```python
from build123d import *

# Parameters (mm, degrees)
F0_W        = 45.5
F0_H        = 83.5
F1_DEPTH    = 52
F2_W        = 34
F2_H        = 72
F3_DEPTH    = 52.001
F5_W        = 15
F5_H        = 2
F6_DEPTH    = 52.001
F8_R        = 2
F10_D       = 4.4
F10_ON_F9_D = 4.4
F10_ON_F4_D = 4.4
F12_DEPTH   = 45.501
F13_W       = 7
F13_H       = 10
F14_DEPTH   = 2.5
F15_W       = 7.7
F15_H       = 31.3
F16_DEPTH   = 2.5


# Not quite as in the source:
# - a feature names something its author has since deleted; it is built from what else it names


with BuildPart() as f1:
    # F0 (on Front) → F1 (new body)
    with BuildSketch(Plane.XZ):
        with Locations((11.25, 30.25)):
            Rectangle(F0_W, F0_H)
    extrude(amount=F1_DEPTH)

    # F2 (on face) → F3 (cut, through all)
    with BuildSketch(Plane.XZ.offset(52)):
        with Locations((17, 36)):
            Rectangle(F2_W, F2_H)
    extrude(amount=-F3_DEPTH, mode=Mode.SUBTRACT)

    # F5 (on face) → F6 (cut, through all)
    with BuildSketch(Plane.XZ.offset(52)):
        with Locations((26.5, -10.5)):
            Rectangle(F5_W, F5_H)
    extrude(amount=-F6_DEPTH, mode=Mode.SUBTRACT)

    # F8
    f8_edges = [f1.edges().sort_by_distance(p)[0] for p in [
        (0, -26, 0),
    ]]
    fillet(f8_edges, radius=F8_R)

    # F10 (through all)
    with Locations(Plane.XY):
        with Locations((26.5, -4.2)):
            Hole(F10_D / 2)

    # F10 on F9 (through all)
    with Locations(Plane(origin=(-11.5, 0, 0), x_dir=(0, -1, 0), z_dir=(-1, 0, 0))):
        with Locations((12.2, 32.3)):
            Hole(F10_ON_F9_D / 2)

    # F10 on F4 (through all)
    with Locations(Plane(origin=(0, 0, -11.5), x_dir=(1, 0, 0), z_dir=(0, 0, -1))):
        with Locations((14.3, 19.8), (14.3, 4.2)):
            Hole(F10_ON_F4_D / 2)

    # F11 (on face) → F12 (cut, through all)
    with BuildSketch(Plane(origin=(-11.5, 0, 0), x_dir=(0, -1, 0), z_dir=(-1, 0, 0))):
        with BuildLine():
            ThreePointArc((47.8, 70), (46.2443650814, 69.3556349186), (45.6, 67.8))
            Line((45.6, 67.8), (45.6, 44.2))
            ThreePointArc((45.6, 44.2), (46.2443650814, 42.6443650814), (47.8, 42))
            ThreePointArc((47.8, 42), (49.3556349186, 42.6443650814), (50, 44.2))
            Line((50, 44.2), (50, 67.8))
            ThreePointArc((50, 67.8), (49.3556349186, 69.3556349186), (47.8, 70))
        make_face()
    extrude(amount=-F12_DEPTH, mode=Mode.SUBTRACT)

    # F13 (on face) → F14 (cut)
    with BuildSketch(Plane.YZ):
        with Locations((-12.2, 32.3)):
            Rectangle(F13_W, F13_H)
    extrude(amount=-F14_DEPTH, mode=Mode.SUBTRACT)

    # F15 (on face) → F16 (cut)
    with BuildSketch(Plane.YZ):
        with Locations((-48.15, 56.35)):
            Rectangle(F15_W, F15_H)
        with BuildLine():
            Line((-50, 44.2), (-50, 67.8))
            ThreePointArc((-50, 67.8), (-47.8, 70), (-45.6, 67.8))
            Line((-45.6, 67.8), (-45.6, 44.2))
            ThreePointArc((-45.6, 44.2), (-47.8, 42), (-50, 44.2))
        make_face(mode=Mode.SUBTRACT)
    extrude(amount=-F16_DEPTH, mode=Mode.SUBTRACT)


solid = f1.part
```
CAD build for the part. Positions are in the model's coordinates, mm. A direction names the side the tool comes from. Coordinates: 2 decimals unless noted, no trailing zeros. Loops run counter-clockwise (first coordinate to the right, second up) from the corner with the lowest first, then second, coordinate; pieces in that order, holes last. Notation, with made-up numbers: (40.5, -20) - (83.5, -20) arc R17 ccw to (83.5, 7) - close; hole circle Ø1 at (-4, 22.25). An arc over 180 degrees is marked (long way). Use CSV: the item, a comma, the result in double quotes. Start each with the question number.
Q1. Cut at A-A, the plane y = -12.2. List the corners of the cut face in (x, z).
Q2. Cut at B-B, the plane x = 26.5. List the corners of the cut face in (y, z), then the cut area to 3 significant figures.
Q3. Probe probe 1 along Y at (x, z) = (14.3, -2.5); probe 2 along Y at (x, z) = (-4, 32); probe 3 along Z at (x, y) = (-4, -12). List the from-to ranges inside material, lowest first. Write a range as from..to.
Q4. Cut at D-D, the plane x = 14.3. List the corners of the cut face in (y, z), then the cut area to 3 significant figures.
Q5. Two-plate mould, pull along Y, no slides. Class faces 1 (the cylindrical face through (0.57, -25.64, 0.6)), 2 (the flat face through (-1, -12, 27.3)), 3 (the flat face through (-2, 0, 21)): +Y half, -Y half, draft (parallel to the pull), parting line (faces both ways), or undercut.
Q6. 3-axis set-ups, long thin cutter, end or side, ignore diameter. For faces 4 (the flat face through (-1, -48, 40.7)), 5 (the flat face through (19, -26, -11)), 6 (the flat face through (-7, -45.6, 56)), 7 (the flat face through (18, -26, 0)), 8 (the flat face through (-1, -15.7, 32)): which of +Z, -Z, +X, -X, +Y, -Y reach the whole face in a straight line?
Q7. Drop flat-ended pins along their axis: P1, Ø12, axis at x = 28.5, y = -20.5, coming from the -Z side; P2, Ø1, axis at x = 4, y = -31.5, coming from the +Z side; P3, Ø1.2, axis at x = -1, y = -46.5, coming from the +Z side. Give the stop position or say it passes through.
Q8. Cut at C-C, the plane z = 32.3. List the corners of the cut face in (x, y), then the cut area to 3 significant figures.
Here are the results:
1,outline,"(-11.5, -11.5) - (19, -11.5) - (19, -9.5) - (34, -9.5) - (34, 0) - (2, 0) arc R2 cw to (0, 2) - (0, 27.3) - (-2.5, 27.3) - (-2.5, 30.1) - (-11.5, 30.1) - close; (-11.5, 34.5) - (-2.5, 34.5) - (-2.5, 37.3) - (0, 37.3) - (0, 72) - (-11.5, 72) - close"
2,outline,"(-52, -9.5) - (-6.4, -9.5) - (-6.4, 0) - (-52, 0) - close; (-2, -9.5) - (0, -9.5) - (0, 0) - (-2, 0) - close"
2,area,"452 mm2"
3,probe 1,"-52..-22, -17.6..-6.4, -2..0"
3,probe 2,"-52..-14.38, -10.02..0"
3,probe 3,"-11.5..30.11, 34.49..72"
4,outline,"(-52, -11.5) - (-22, -11.5) - (-22, 0) - (-52, 0) - close; (-17.6, -11.5) - (-6.4, -11.5) - (-6.4, 0) - (-17.6, 0) - close; (-2, -11.5) - (0, -11.5) - (0, 0) - (-2, 0) - close"
4,area,"497 mm2"
5,face 1,"draft"
5,face 2,"undercut"
5,face 3,"+Y half"
6,face 4,"+Z, +X, -Y"
6,face 5,"-Z, +X, +Y, -Y"
6,face 6,"+X, -X"
6,face 7,"+Z, +X, +Y, -Y"
6,face 8,"+X"
7,P1,"z = -9.5"
7,P2,"z = 0"
7,P3,"z = 40.7"
8,outline,"(-11.5, -52) - (0, -52) - (0, -15.7) - (-2.5, -15.7) - (-2.5, -14.4) - (-11.5, -14.4) - close; (-11.5, -10) - (-2.5, -10) - (-2.5, -8.7) - (0, -8.7) - (0, 0) - (-11.5, 0) - close"
8,area,"541 mm2"
